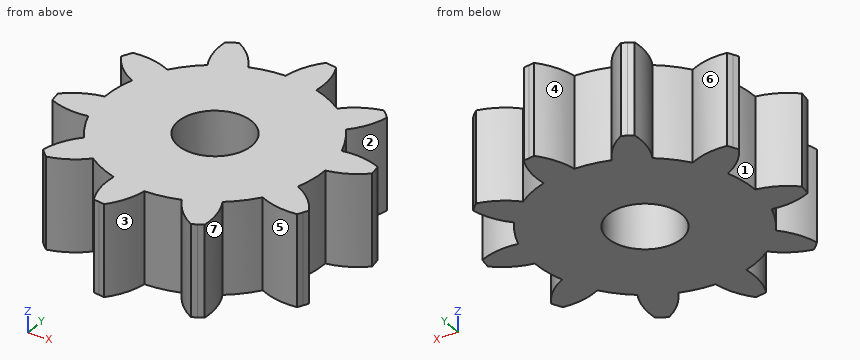
from build123d import *

# Parameters (mm, degrees)
F1_DEPTH = 2.5
F2_R     = 1
F3_DEPTH = 2.501


with BuildPart() as f1:
    # F0 (on Top) → F1 (new body)
    with BuildSketch(Plane.XY):
        with BuildLine():
            ThreePointArc((2.85317, 0.927051), (2.67302, 1.361971), (2.427051, 1.763356))
            ThreePointArc((2.427051, 1.763356), (2.752898, 2.200719), (2.938951, 2.713405))
            ThreePointArc((2.938951, 2.713405), (2.884263, 2.771467), (2.828427, 2.828427))
            ThreePointArc((2.828427, 2.828427), (2.771467, 2.884263), (2.713405, 2.938951))
            ThreePointArc((2.713405, 2.938951), (2.200719, 2.752898), (1.763356, 2.427051))
            ThreePointArc((1.763356, 2.427051), (1.361971, 2.67302), (0.927051, 2.85317))
            ThreePointArc((0.927051, 2.85317), (0.933592, 3.398532), (0.782762, 3.922663))
            ThreePointArc((0.782762, 3.922663), (0.70439, 3.937491), (0.625738, 3.950753))
            ThreePointArc((0.625738, 3.950753), (0.546837, 3.962445), (0.467718, 3.972561))
            ThreePointArc((0.467718, 3.972561), (0.162306, 3.520692), (0, 3))
            ThreePointArc((0, 3), (-0.469303, 2.963065), (-0.927051, 2.85317))
            ThreePointArc((-0.927051, 2.85317), (-1.242315, 3.298221), (-1.672415, 3.633597))
            ThreePointArc((-1.672415, 3.633597), (-1.744535, 3.599527), (-1.815962, 3.564026))
            ThreePointArc((-1.815962, 3.564026), (-1.886666, 3.527108), (-1.956621, 3.488787))
            ThreePointArc((-1.956621, 3.488787), (-1.938103, 2.9437), (-1.763356, 2.427051))
            ThreePointArc((-1.763356, 2.427051), (-2.12132, 2.12132), (-2.427051, 1.763356))
            ThreePointArc((-2.427051, 1.763356), (-2.9437, 1.938103), (-3.488787, 1.956621))
            ThreePointArc((-3.488787, 1.956621), (-3.527108, 1.886666), (-3.564026, 1.815962))
            ThreePointArc((-3.564026, 1.815962), (-3.599527, 1.744535), (-3.633597, 1.672415))
            ThreePointArc((-3.633597, 1.672415), (-3.298221, 1.242315), (-2.85317, 0.927051))
            ThreePointArc((-2.85317, 0.927051), (-2.963065, 0.469303), (-3, 0))
            ThreePointArc((-3, 0), (-3.520692, -0.162306), (-3.972561, -0.467718))
            ThreePointArc((-3.972561, -0.467718), (-3.962445, -0.546837), (-3.950753, -0.625738))
            ThreePointArc((-3.950753, -0.625738), (-3.937491, -0.70439), (-3.922663, -0.782762))
            ThreePointArc((-3.922663, -0.782762), (-3.398532, -0.933592), (-2.85317, -0.927051))
            ThreePointArc((-2.85317, -0.927051), (-2.67302, -1.361971), (-2.427051, -1.763356))
            ThreePointArc((-2.427051, -1.763356), (-2.752898, -2.200719), (-2.938951, -2.713405))
            ThreePointArc((-2.938951, -2.713405), (-2.884263, -2.771467), (-2.828427, -2.828427))
            ThreePointArc((-2.828427, -2.828427), (-2.771467, -2.884263), (-2.713405, -2.938951))
            ThreePointArc((-2.713405, -2.938951), (-2.200719, -2.752898), (-1.763356, -2.427051))
            ThreePointArc((-1.763356, -2.427051), (-1.361971, -2.67302), (-0.927051, -2.85317))
            ThreePointArc((-0.927051, -2.85317), (-0.933592, -3.398532), (-0.782762, -3.922663))
            ThreePointArc((-0.782762, -3.922663), (-0.70439, -3.937491), (-0.625738, -3.950753))
            ThreePointArc((-0.625738, -3.950753), (-0.546837, -3.962445), (-0.467718, -3.972561))
            ThreePointArc((-0.467718, -3.972561), (-0.162306, -3.520692), (0, -3))
            ThreePointArc((0, -3), (0.469303, -2.963065), (0.927051, -2.85317))
            ThreePointArc((0.927051, -2.85317), (1.242315, -3.298221), (1.672415, -3.633597))
            ThreePointArc((1.672415, -3.633597), (1.744535, -3.599527), (1.815962, -3.564026))
            ThreePointArc((1.815962, -3.564026), (1.886666, -3.527108), (1.956621, -3.488787))
            ThreePointArc((1.956621, -3.488787), (1.938103, -2.9437), (1.763356, -2.427051))
            ThreePointArc((1.763356, -2.427051), (2.12132, -2.12132), (2.427051, -1.763356))
            ThreePointArc((2.427051, -1.763356), (2.9437, -1.938103), (3.488787, -1.956621))
            ThreePointArc((3.488787, -1.956621), (3.527108, -1.886666), (3.564026, -1.815962))
            ThreePointArc((3.564026, -1.815962), (3.599527, -1.744535), (3.633597, -1.672415))
            ThreePointArc((3.633597, -1.672415), (3.298221, -1.242315), (2.85317, -0.927051))
            ThreePointArc((2.85317, -0.927051), (2.963065, -0.469303), (3, 0))
            ThreePointArc((3, 0), (3.520692, 0.162306), (3.972561, 0.467718))
            ThreePointArc((3.972561, 0.467718), (3.962445, 0.546837), (3.950753, 0.625738))
            ThreePointArc((3.950753, 0.625738), (3.937491, 0.70439), (3.922663, 0.782762))
            ThreePointArc((3.922663, 0.782762), (3.398532, 0.933592), (2.85317, 0.927051))
        make_face()
    extrude(amount=F1_DEPTH)

    # F2 (on face) → F3 (cut, through all)
    with BuildSketch(Plane.XY.offset(2.5)):
        Circle(F2_R)
    extrude(amount=-F3_DEPTH, mode=Mode.SUBTRACT)


solid = f1.part
The model under review builds one solid part; all positions refer to its coordinate system, in mm. Face numbers are marked on the shaded views. A direction names the side the tool comes from. Round coordinates to 2 decimals unless told otherwise and drop trailing zeros. Loops run counter-clockwise (first coordinate to the right, second up) from the corner with the lowest first, then second, coordinate; pieces in that order, holes last. Notation, with made-up numbers: (49, -32.75) -> (105, -32.75) arc R10 cw to (105, -23.75) -> close; hole circle Ø7 at (39.25, 89.5). An arc over 180 degrees is marked (long way). One line per question, with ' | ' between items. Start each with the question number.
Item 1: Draft analysis for pull direction Y (two halves, no side actions). For the marked faces 5, 6 and 7, state which applies: +Y half, -Y half, draft (parallel to the pull), parting line (faces both ways), or undercut.
Item 2: For pin 1 (1.2 mm diameter, centred on x = 0, y = 0, fed in from -Z), flat-tipped, find the tip position at first contact; note if it passes through.
Item 3: Add section A-A, the plane y = 3.25. Write out the cut boundary in (x, z), then the cut area to 3 significant figures.
Item 4: Add section B-B, the plane x = 2.25. Write out the cut boundary in (y, z).
Item 5: Machinability: for the marked faces 1, 2, 3 and 4, which of the approach directions +Z, -Z, +X, -X, +Y, -Y give a long, thin tool a straight path to every point of the face, cutting with its end or side? Answer none if there is none.
Item 6: Wall thickness on line 1 along Y through (x, z) = (3.25, 0.5); line 2 along X through (y, z) = (0.5, 1.9); line 3 along Y through (x, z) = (-3.25, 2): over which ranges is each line inside the solid? List them lowest first. Write a range as [from, to].
Return value:
1) face 5: -Y half | face 6: +Y half | face 7: undercut
2) pin 1: passes through
3) outline: (-1.97, 0) -> (-1.2, 0) -> (-1.2, 2.5) -> (-1.97, 2.5) -> close; (0.06, 0) -> (0.95, 0) -> (0.95, 2.5) -> (0.06, 2.5) -> close | area: 4.15 mm2
4) outline: (-1.98, 0) -> (2.78, 0) -> (2.78, 2.5) -> (-1.98, 2.5) -> close
5) face 1: +Z, -Z, -X | face 2: +Z, -Z, +X | face 3: +Z, -Z, -Y | face 4: +Z, -Z, +Y
6) line 1: y = [-1.97, -1.2], [0.06, 0.95] | line 2: x = [-2.96, -0.87], [0.87, 3.97] | line 3: y = [-0.95, -0.06], [1.2, 1.97]
